Geometry check sheet. Reference: the model listing, model coordinates, mm. Face numbers are marked on the shaded views. Round coordinates to 2 decimals unless told otherwise and drop trailing zeros. Loops run counter-clockwise (first coordinate to the right, second up) from the corner with the lowest first, then second, coordinate; pieces in that order, holes last. Notation, with made-up numbers: M 34.5,42.5 L 64.5,42.5 A14 ccw 64.5,55.5 Z; hole C 15,41 d4. An arc over 180 degrees is marked long. Use one line per item in the form item = value. Start each with the question number.
1. Material ranges on line 1 (X direction, y = 64.5, z = 15.5); line 2 (Y direction, x = -28.5, z = 26); line 3 (Y direction, x = 43.5, z = 8), recorded low to high.
2. Draft check along Z on the marked faces 1, 2, 3 and 4. Enter one of: pulls with the +Z half, pulls with the -Z half, needs draft (parallel to the pull), parting line crosses it, or undercut.
3. Cross-section at D-D (x = -41). Record the boundary of the cut face in (y, z).
4. Cross-section at A-A (y = 67). Record the boundary of the cut face in (x, z).
5. Cross-section at C-C (x = -8.5). Record the boundary of the cut face in (y, z), then the cut area to 3 significant figures.
6. Go/stop test with flat-tipped pins: pin 1 (5.5 mm diameter, centred on x = 42.2, z = -4.34, fed in from -Y); pin 2 (6 mm diameter, centred on x = 8.5, z = -2.5, fed in from +Y); pin 3 (2.5 mm diameter, centred on x = -23, z = 17.5, fed in from +Y). Record where each tip stops, or that it passes through.
7. Cross-section at B-B (x = -27.5). Record the boundary of the cut face in (y, z), then the cut area to 3 significant figures.
```python
from build123d import *

# Parameters (mm, degrees)
SKETCH_1_W           = 95
SKETCH_1_H           = 61.7
EXTRUDE_1_DEPTH      = 93
SKETCH_3_OUTSIDE_W   = 126.312
SKETCH_3_OUTSIDE_H   = 93.012
SKETCH_3_OUTSIDE_W_2 = 95
SKETCH_3_OUTSIDE_H_2 = 19.4
CUT_EXTRUDE_1_DEPTH  = 1
SKETCH_4_R           = 3
CUT_EXTRUDE_2_DEPTH  = 3
SKETCH_5_W           = 95
SKETCH_5_H           = 8
CUT_EXTRUDE_3_DEPTH  = 6
SKETCH_6_W           = 95
SKETCH_6_H           = 19.4
CUT_EXTRUDE_4_DEPTH  = 2
SKETCH_7_R           = 3
CUT_EXTRUDE_5_DEPTH  = 121.528585821


with BuildPart() as part:
    # 草图1 → 凸台-拉伸1 (new body)
    with BuildSketch(Plane(origin=(0, 0, 0), x_dir=(1, 0, 0), z_dir=(0, 1, 0))):
        Rectangle(SKETCH_1_W, SKETCH_1_H)
    extrude(amount=EXTRUDE_1_DEPTH)

    # 草图3 outside → 切除-拉伸1 (cut)
    with BuildSketch(Plane(origin=(0, 93, 0), x_dir=(1, 0, 0), z_dir=(0, 1, 0))):
        Rectangle(SKETCH_3_OUTSIDE_W, SKETCH_3_OUTSIDE_H)
        Rectangle(SKETCH_3_OUTSIDE_W_2, SKETCH_3_OUTSIDE_H_2, mode=Mode.SUBTRACT)
    extrude(amount=-CUT_EXTRUDE_1_DEPTH, mode=Mode.SUBTRACT)

    # 草图4 → 切除-拉伸2 (cut)
    with BuildSketch(Plane(origin=(0, 93, 0), x_dir=(1, 0, 0), z_dir=(0, 1, 0))):
        with Locations(Location((-42.196054271, -4.338164654, 0), (0, 0, 270))):
            Circle(SKETCH_4_R)
        with Locations(Location((42.196054271, 4.338164654, 0), (0, 0, 270))):
            Circle(SKETCH_4_R)
    extrude(amount=-CUT_EXTRUDE_2_DEPTH, mode=Mode.SUBTRACT)

    # 草图5 → 切除-拉伸3 (cut)
    with BuildSketch(Plane(origin=(0, 92, 0), x_dir=(1, 0, 0), z_dir=(0, 1, 0))):
        with Locations((0, -18.2)):
            Rectangle(SKETCH_5_W, SKETCH_5_H)
        with Locations((0, 18.2)):
            Rectangle(SKETCH_5_W, SKETCH_5_H)
    extrude(amount=-CUT_EXTRUDE_3_DEPTH, mode=Mode.SUBTRACT)

    # 草图6 → 切除-拉伸4 (cut)
    with BuildSketch(Plane(origin=(0, 93, 0), x_dir=(1, 0, 0), z_dir=(0, 1, 0))):
        Rectangle(SKETCH_6_W, SKETCH_6_H)
    extrude(amount=-CUT_EXTRUDE_4_DEPTH, mode=Mode.SUBTRACT)

    # 草图7 → 切除-拉伸5 (cut, through all)
    with BuildSketch(Plane.XY.offset(30.85)):
        with Locations((-27.5, 67)):
            Circle(SKETCH_7_R)
        with Locations(Location((27.5, 67, 0), (0, 0, 180))):
            Circle(SKETCH_7_R)
    extrude(amount=-CUT_EXTRUDE_5_DEPTH, mode=Mode.SUBTRACT)


solid = part.part
```
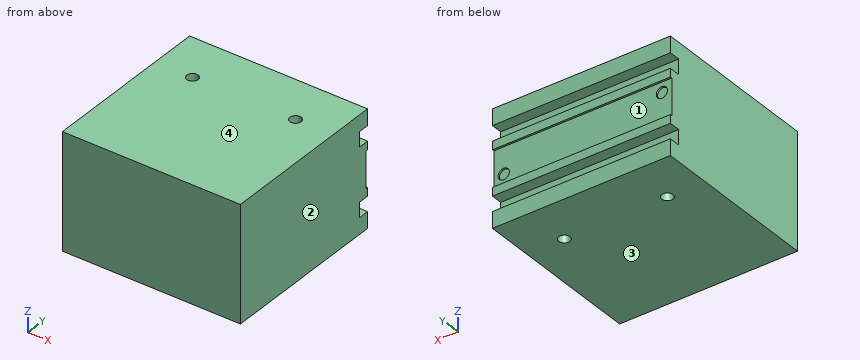
Reported:
q1.line_1 = -47.5 to -29.16, -25.84 to 25.84, 29.16 to 47.5
q1.line_2 = 0 to 64.17, 69.83 to 92
q1.line_3 = 0 to 91
q2.face_1 = undercut
q2.face_2 = needs draft
q2.face_3 = pulls with the -Z half
q2.face_4 = pulls with the +Z half
q3.outline = M 0,-30.85 L 92,-30.85 L 92,-22.2 L 86,-22.2 L 86,-14.2 L 92,-14.2 L 92,-9.7 L 91,-9.7 L 91,1.59 L 90,1.59 L 90,7.09 L 91,7.09 L 91,9.7 L 92,9.7 L 92,14.2 L 86,14.2 L 86,22.2 L 92,22.2 L 92,30.85 L 0,30.85 Z
q4.outline = M -47.5,-30.85 L -30.5,-30.85 L -30.5,30.85 L -47.5,30.85 Z; M -24.5,-30.85 L 24.5,-30.85 L 24.5,30.85 L -24.5,30.85 Z; M 30.5,-30.85 L 47.5,-30.85 L 47.5,30.85 L 30.5,30.85 Z
q5.outline = M 0,-30.85 L 92,-30.85 L 92,-22.2 L 86,-22.2 L 86,-14.2 L 92,-14.2 L 92,-9.7 L 91,-9.7 L 91,9.7 L 92,9.7 L 92,14.2 L 86,14.2 L 86,22.2 L 92,22.2 L 92,30.85 L 0,30.85 Z
q5.area = 5,560 mm²
q6.pin_1 = 0
q6.pin_2 = 91
q6.pin_3 = 86
q7.outline = M 0,-30.85 L 64,-30.85 L 64,30.85 L 0,30.85 Z; M 70,-30.85 L 92,-30.85 L 92,-22.2 L 86,-22.2 L 86,-14.2 L 92,-14.2 L 92,-9.7 L 91,-9.7 L 91,9.7 L 92,9.7 L 92,14.2 L 86,14.2 L 86,22.2 L 92,22.2 L 92,30.85 L 70,30.85 Z
q7.area = 5,190 mm²
